Read the model definition and answer for the solid it produces. Units are mm, in the model's axes. Face numbers are marked on the shaded views. A direction names the side the tool comes from. Give positions to 0.01 mm unless a question says otherwise; leave off trailing zeros. Loops run counter-clockwise (first coordinate to the right, second up) from the corner with the lowest first, then second, coordinate; pieces in that order, holes last.
(1) Find section D-D, the plane x = 96. Write down the section's boundary in (y, z), then the cut area to 3 significant figures.
(2) Find section A-A, the plane z = 0. Write down the section's boundary in (x, y), then the cut area to 3 significant figures.
(3) Which of the six approach directions +Z, -Z, +X, -X, +Y, -Y give full straight-line access (tool end or side, diameter ignored) to the marked faces 1, 2 and 3?
(4) Find section C-C, the plane x = 15. Write down the section's boundary in (y, z), then the cut area to 3 significant figures.
(5) Determine the mould class of the marked faces 4 and 5 for opening direction Z: pulls with the +Z half, pulls with the -Z half, needs draft (parallel to the pull), parting line crosses it, or undercut.
(6) Find section B-B, the plane y = 0. Write down the section's boundary in (x, z), then the cut area to 3 significant figures.
(7) Straight lines are drawn through the part: probe 1 along X at (y, z) = (-8, 0); probe 2 along Z at (x, y) = (15, 0.25); probe 3 along X at (y, z) = (-13, -7). For each, find the intervals that lie inside material, in ascending order.
(8) Each of these flat-tipped pins is pushed along its axis until it touches: P1, Ø6, axis at x = 28, z = -6, coming from the -Y side; P2, Ø4, axis at x = 48.5, z = -1, coming from the +Y side; P3, Ø6, axis at x = 105.5, z = -6.5, coming from the -Y side; P4, Ø3.5, axis at x = 15, z = 0, coming from the +Y side. Where does it stop, or does it pass through?
```python
from build123d import *

# Parameters (mm, degrees)
SKETCH_1_R          = 10
EXTRUDE_1_DEPTH     = 30
SKETCH_2_R          = 15
EXTRUDE_2_DEPTH     = 50
SKETCH_3_R          = 12
EXTRUDE_3_DEPTH     = 40
CUT_EXTRUDE_1_DEPTH = 4
SKETCH_5_R          = 3
CUT_EXTRUDE_2_DEPTH = 121


with BuildPart() as part:
    # 草图1 → 凸台-拉伸1 (new body)
    with BuildSketch(Plane(origin=(0, 0, 0), x_dir=(0, 0, -1), z_dir=(1, 0, 0))):
        Circle(SKETCH_1_R)
    extrude(amount=EXTRUDE_1_DEPTH)

    # 草图2 → 凸台-拉伸2 (add)
    with BuildSketch(Plane(origin=(30, 0, 0), x_dir=(0, 0, -1), z_dir=(1, 0, 0))):
        Circle(SKETCH_2_R)
    extrude(amount=EXTRUDE_2_DEPTH)

    # 草图3 → 凸台-拉伸3 (add)
    with BuildSketch(Plane(origin=(80, 0, 0), x_dir=(0, 0, -1), z_dir=(1, 0, 0))):
        Circle(SKETCH_3_R)
    extrude(amount=EXTRUDE_3_DEPTH)

    # 草图4 → 切除-拉伸1 (cut)
    with BuildSketch(Plane(origin=(0, 15, 0), x_dir=(1, 0, 0), z_dir=(0, 1, 0))):
        with BuildLine():
            Line((44, 4), (66, 4))
            ThreePointArc((66, 4), (70, 0), (66, -4))
            Line((66, -4), (44, -4))
            ThreePointArc((44, -4), (40, 0), (44, 4))
        make_face()
    extrude(amount=-CUT_EXTRUDE_1_DEPTH, mode=Mode.SUBTRACT)

    # 草图5 → 切除-拉伸2 (cut, symmetric)
    with BuildSketch(Plane(origin=(0, 0, 0), x_dir=(1, 0, 0), z_dir=(0, 1, 0))):
        with Locations(Location((15, 0, 0), (0, 0, 270))):
            Circle(SKETCH_5_R)
    extrude(amount=CUT_EXTRUDE_2_DEPTH, both=True, mode=Mode.SUBTRACT)


solid = part.part
```
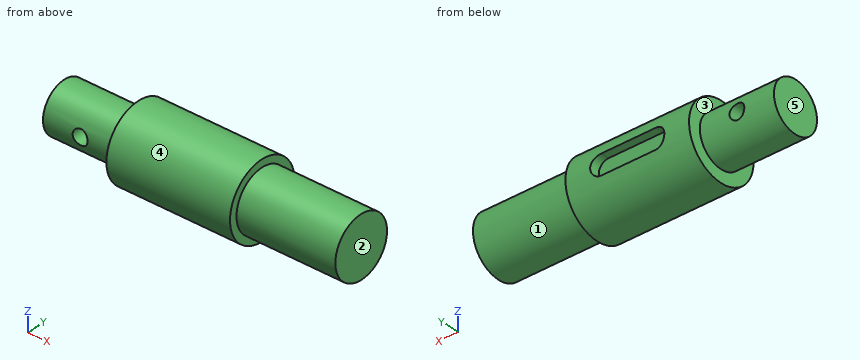
Entries:
1. outline: circle Ø24 at (0, 0)
1. area: 452 mm2
2. outline: (0, -10) - (12, -10) - (12, 10) - (0, 10) - close; (18, -10) - (30, -10) - (30, -15) - (80, -15) - (80, -12) - (120, -12) - (120, 12) - (80, 12) - (80, 15) - (70, 15) - (70, 11) - (40, 11) - (40, 15) - (30, 15) - (30, 10) - (18, 10) - close
2. area: 2,820 mm2
3. face 1: +X
3. face 2: +Z, -Z, +X, +Y, -Y
3. face 3: -X
4. outline: (-9.54, -3) arc R10 ccw to (9.54, -3) - close; (-9.54, 3) - (9.54, 3) arc R10 ccw to start
4. area: 196 mm2
5. face 4: parting line crosses it
5. face 5: needs draft
6. outline: (0, -10) - (30, -10) - (30, -15) - (80, -15) - (80, -12) - (120, -12) - (120, 12) - (80, 12) - (80, 15) - (30, 15) - (30, 10) - (0, 10) - close; hole circle Ø6 at (15, 0)
6. area: 3,030 mm2
7. probe 1: x = 0 to 12, 18 to 120
7. probe 2: z = -10 to -3, 3 to 10
7. probe 3: x = 30 to 80
8. P1: stops at y = -14.52
8. P2: stops at y = 11
8. P3: stops at y = -11.48
8. P4: passes through
